Read the model definition and answer for the solid it produces. Units are mm, in the model's axes. A direction names the side the tool comes from. Coordinates: 2 decimals unless noted, no trailing zeros. Order: outer loops, then holes, each group sorted by start corner. A loop starts at its lowest first (then second) coordinate and runs counter-clockwise, first axis right, second up. Notation, with made-up numbers: (-12, 51) -> (45, 51) arc R25 ccw to (45, 76) -> close; hole circle Ø10 at (-26.75, 15). An arc over 180 degrees is marked (long way). Use CSV: the item, a comma, the result in double quotes.
Autodesk Inventor part; units mm, degrees
ref_plane "YZ Plane" through (0, 0, 0) normal (1, 0, 0) x (0, 1, 0)
ref_plane "XZ Plane" through (0, 0, 0) normal (0, 1, 0) x (-1, 0, 0)
ref_plane "XY Plane" through (0, 0, 0) normal (0, 0, 1) x (1, 0, 0)
sketch "Sketch1" plane through (0, 0, 0) normal (0, 1, 0) x (-1, 0, 0)
  line L0 (0, 0) -> (3.175, 0)
  line L1 (5.3594, -2.3876) -> (5.3594, -3.175)
  line L2 (5.3594, -3.175) -> (3.175, -3.175)
  line L3 (3.175, -3.175) -> (3.175, -28.575)
  line L4 (3.175, -28.575) -> (0, -28.575)
  line L5 (0, -28.575) -> (0, 0)
  arc A0 (5.3594, -2.3876) -> (3.175, 0) centre (0.0087, -5.0899) ccw
  dimension "d0" = 3.175
  dimension "d1" = 5.3594
  dimension "d2" = 0.7874
  dimension "d3" = 3.175
  dimension "d8" = 3.175
  dimension "d9" = 5.9944
  dimension "d20" = 25.4
revolve "Revolution1" add sketch "Sketch1" angle 360 about axis through (0, 0, -28.575) along (0, 0, 1)
chamfer "Chamfer1" distance 0.762 angle 45 1 edges at (3.175, 0, -28.575)
sketch "Sketch2" plane through (0, 0, 0) normal (0, 0, 1) x (1, 0, 0)
  line L0 (1.9844, 0) -> (0.9922, -1.7185)
  line L1 (0.9922, -1.7185) -> (-0.9922, -1.7185)
  line L2 (-0.9922, -1.7185) -> (-1.9844, 0)
  line L3 (-1.9844, 0) -> (-0.9922, 1.7185)
  line L4 (-0.9922, 1.7185) -> (0.9922, 1.7185)
  line L5 (0.9922, 1.7185) -> (1.9844, 0)
  point P0 (0, 0)
  point P1 (0, 0)
  dimension "d14" = 3.9688
extrude "Extrusion1" cut sketch "Sketch2" against normal blind 2.8194
thread "Thread1"
properties part number "Axle Peg"
Item 1: Each of these flat-tipped pins is pushed along its axis until it touches: P1, Ø2.5, axis at x = 0, y = 0, coming from the +Z side; P2, Ø1, axis at x = -2, z = -9.5, coming from the +Y side; P3, Ø0.6, axis at x = 0, z = -2, coming from the -Y side. Where does it stop, or does it pass through?
Return value:
P1,"stops at z = -2.82"
P2,"stops at y = 2.8"
P3,"stops at y = -5.31"
Item 2: The mould has two halves that part along X. Classify faces 1 (the cylindrical face through (0.69, -3.1, -15.67)), 2 (the flat face through (0, 1.718, -1)), 3 (the flat face through (0, 0, -28.575)): +X half, -X half, draft (parallel to the pull), parting line (faces both ways), or undercut.
Return value:
face 1,"parting line"
face 2,"undercut"
face 3,"draft"
Item 3: Find section A-A, the plane z = -4.25. Give the vertices of the cut face in (x, y) (3 decimals), then the cut area to 3 significant figures.
Return value:
outline,"circle Ø6.35 at (0, 0)"
area,"31.7 mm^2"
Item 4: Straight lines are drawn through the part: line 1 along Z through (x, y) = (-1.25, 0) (3 decimals); line 2 along Y through (x, z) = (0, -21) (3 decimals); line 3 along Z through (x, y) = (5, 0) (3 decimals). For each, find the intervals that lie inside material, in ascending order.
Return value:
line 1,"z = -28.575 to -2.819"
line 2,"y = -3.175 to 3.175"
line 3,"z = -3.175 to -1.77"
Item 5: A tool of negligible diameter and unlimited length cuts with its end or side. For faces 4 (the flat face through (-1.4, 1.4, 0)), 5 (the flat face through (0, 0, -2.819)), 6 (the flat face through (0.1, 3.5, -3.175)), from which of +Z, -Z, +X, -X, +Y, -Y can it reach the whole face along a straight path? Write none if from no direction.
Return value:
face 4,"+Z, +X, -X, +Y, -Y"
face 5,"+Z"
face 6,"-Z"
